For this review, take the finished solid that the model builds, in its own axes (mm). Face numbers are marked on the shaded views. A direction names the side the tool comes from. Coordinates: 2 decimals unless noted, no trailing zeros. Loops run counter-clockwise (first coordinate to the right, second up) from the corner with the lowest first, then second, coordinate; pieces in that order, holes last. Notation, with made-up numbers: (38, 39) -> (82, 39) arc R8 ccw to (82, 43) -> close; hole circle Ø1 at (-3, 48). An arc over 180 degrees is marked (long way). Answer in a Markdown table with one row per item.
from build123d import *

# Parameters (mm, degrees)
EXTRUSION1_DEPTH        = 23.5
EXTRUSION2_DEPTH        = 5.5
EXTRUSION3_DEPTH        = 5.5
ENL_V_MAT_EXTRU_1_DEPTH = 0.5


with BuildPart() as part:
    # Esquisse1 → Extrusion1 (new body)
    with BuildSketch(Plane.XY):
        with BuildLine():
            Line((-8.839098079, -7.6), (3.170901921, -7.6))
            ThreePointArc((3.170901921, -7.6), (7.767095998, -9.503805922), (9.670901921, -14.1))
            Line((9.670901921, -14.1), (9.670901921, -14.11))
            ThreePointArc((9.670901921, -14.11), (7.770024931, -18.69912301), (3.180901921, -20.6))
            Line((3.180901921, -20.6), (-8.829098079, -20.6))
            ThreePointArc((-8.829098079, -20.6), (-13.425292157, -18.696194078), (-15.329098079, -14.1))
            Line((-15.329098079, -14.1), (-15.329098079, -14.09))
            ThreePointArc((-15.329098079, -14.09), (-13.428221089, -9.50087699), (-8.839098079, -7.6))
        make_face()
    extrude(amount=-EXTRUSION1_DEPTH)

    # Esquisse2 → Extrusion2 (add, symmetric)
    with BuildSketch(Plane(origin=(-3, 0, 0), x_dir=(0, 0, -1), z_dir=(1, 0, 0))):
        Polygon((0, -18.324724565), (0, -11.607872713), (-0.824207274, -5.6), (-1.328890469, -5.6), (-0.5, -11.64200981), (-0.5, -18.324724565), align=None)
    extrude(amount=EXTRUSION2_DEPTH, both=True)

    # Esquisse3 → Extrusion3 (add, symmetric)
    with BuildSketch(Plane(origin=(-3, 0, 0), x_dir=(0, 0, -1), z_dir=(1, 0, 0))):
        Polygon((23.5, -18.324724565), (24, -18.324724565), (24, -14.11), (26.890994991, -5.6), (26.362930623, -5.6), (23.5, -14.027389076), align=None)
    extrude(amount=EXTRUSION3_DEPTH, both=True)

    # Esquisse4 → Enlèv. mat.-Extru.1 (cut)
    with BuildSketch(Plane(origin=(0, -8.769547771, -25.814244494), x_dir=(-1, 0, 0), z_dir=(0, -0.32166286073299966, -0.9468542675750388))):
        Polygon((0.645397002, 3.83477814), (-2.5, -2.321461893), (-3.257578705, -2.321461893), (-3.257578705, 4.719989125), (9.257578705, 4.719989125), (9.257578705, -2.321461893), (8.5, -2.321461893), (5.354602998, 3.83477814), align=None)
    extrude(amount=-ENL_V_MAT_EXTRU_1_DEPTH, mode=Mode.SUBTRACT)


solid = part.part
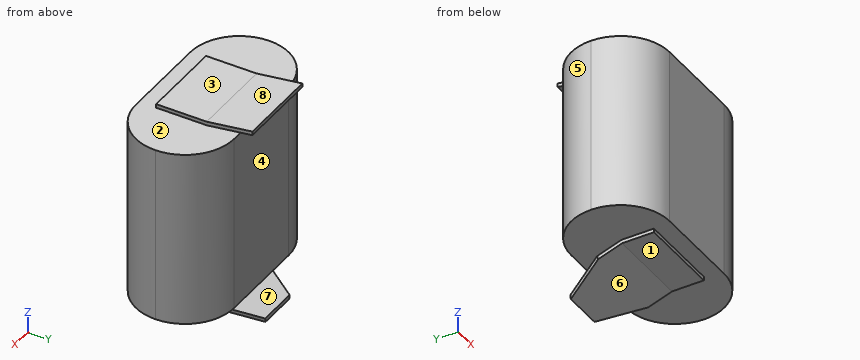
Item 1: Take a section at C-C, the plane x = -5.25. State the section outline as (y, z) points, and give its area (3 significant figures).
Worked answers:
| item | result |
|---|---|
| outline | (-20.6, -23.5) -> (-18.32, -23.5) -> (-18.32, -24) -> (-14.11, -24) -> (-5.6, -26.89) -> (-5.6, -26.36) -> (-14.03, -23.5) -> (-7.6, -23.5) -> (-7.6, 0) -> (-11.61, 0) -> (-5.6, 0.82) -> (-5.6, 1.33) -> (-11.64, 0.5) -> (-18.32, 0.5) -> (-18.32, 0) -> (-20.6, 0) -> close |
| area | 318 mm² |
Item 2: Take a section at A-A, the plane y = -9.5. State the section outline as (x, z) points, and give its area (3 significant figures).
Worked answers:
| item | result |
|---|---|
| outline | (-13.43, -23.5) -> (7.76, -23.5) -> (7.76, 0) -> (-13.43, 0) -> close; (-8.5, 0.29) -> (2.5, 0.29) -> (2.5, 0.79) -> (-8.5, 0.79) -> close; (-7.79, -25.04) -> (-7.71, -25.57) -> (1.71, -25.57) -> (1.79, -25.04) -> close |
| area | 509 mm² |
Item 3: For the marked faces 1, 2, 3 and 4, list the 3-axis set-ups (+Z, -Z, +X, -X, +Y, -Y) from which the entire face can be reached by the end or side of a thin tool; tool diameter is ignored.
Worked answers:
| item | result |
|---|---|
| face 1 | -Z, +X, -X, -Y |
| face 2 | none |
| face 3 | +Z, +X, -X, -Y |
| face 4 | +X, -X, +Y |
Item 4: Take a section at D-D, the plane y = -13.25. State the section outline as (x, z) points.
Worked answers:
| item | result |
|---|---|
| outline | (-15.27, -23.5) -> (9.62, -23.5) -> (9.62, 0) -> (2.5, 0) -> (2.5, 0.5) -> (-8.5, 0.5) -> (-8.5, 0) -> (-15.27, 0) -> close; (-8.5, -24.29) -> (2.5, -24.29) -> (2.5, -23.76) -> (-8.5, -23.76) -> close |
Item 5: Insertion check: pin 1 (1.7 mm diameter, centred on y = -15.5, z = -24, fed in from +X); pin 2 (4 mm diameter, centred on x = 5.5, z = -3.5, fed in from +Y); pin 3 (0.6 mm diameter, centred on x = -2.5, z = 0.5, fed in from -Y). Each pin has a flat end and moves straight along its axis. Give the tip position at first contact, or say it passes through.
Worked answers:
| item | result |
|---|---|
| pin 1 | x = 9.63 |
| pin 2 | y = -7.61 |
| pin 3 | y = -18.32 |
Item 6: For L1, parallel to Z at x = -2.75, y = -10.25; L2, parallel to Z at x = -2, y = -8.75; L3, parallel to Y at x = 2.75, z = -7, list the stretches that pass through material, from the lowest coordinate up.
Worked answers:
| item | result |
|---|---|
| L1 | -25.31 to -24.78, -23.5 to 0, 0.19 to 0.69 |
| L2 | -25.82 to -25.29, -23.5 to 0, 0.39 to 0.9 |
| L3 | -20.6 to -7.6 |
Item 7: The part is to be moulded in two halves that separate along Z. For the marked faces 5, 6, 7 and 8, say which applies: +Z half, -Z half, draft (parallel to the pull), parting line (faces both ways), or undercut.
Worked answers:
| item | result |
|---|---|
| face 5 | draft |
| face 6 | -Z half |
| face 7 | undercut |
| face 8 | +Z half |
